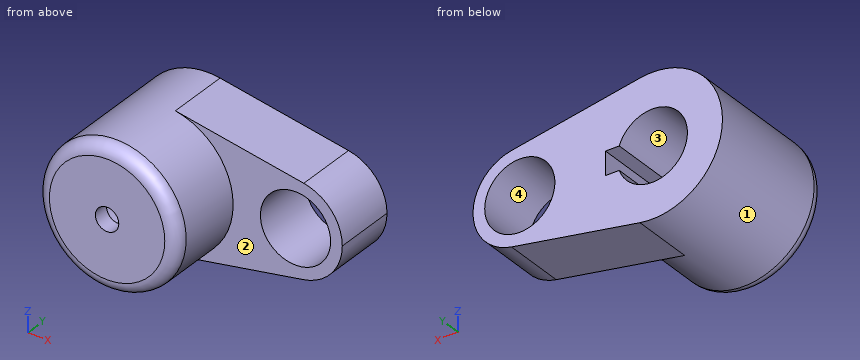
```python
from build123d import *

# Parameters (mm, degrees)
F0_R     = 14.2875
F1_DEPTH = 25.4
F2_DEPTH = 50.8
F3_R     = 28.575
F3_R_2   = 4.7625
F4_DEPTH = 6.35
F5_R     = 5.08


with BuildPart() as f1:
    # F0 (on Front) → F1 (new body)
    with BuildSketch(Plane.XZ):
        with BuildLine():
            ThreePointArc((5.0426470588, -28.1265414802), (21.9160245563, -18.3362616868), (28.575, 0))
            ThreePointArc((28.575, 0), (21.9160245563, 18.3362616868), (5.0426470588, 28.1265414802))
            ThreePointArc((5.0426470588, 28.1265414802), (-28.575, 0), (5.0426470588, -28.1265414802))
        make_face()
        with BuildLine():
            ThreePointArc((-13.4703841816, 4.7625), (0, 14.2875), (13.4703841816, 4.7625))
            Line((13.4703841816, 4.7625), (19.05, 4.7625))
            Line((19.05, 4.7625), (19.05, -4.7625))
            Line((19.05, -4.7625), (13.4703841816, -4.7625))
            ThreePointArc((13.4703841816, -4.7625), (0, -14.2875), (-13.4703841816, -4.7625))
            Line((-13.4703841816, -4.7625), (-19.05, -4.7625))
            Line((-19.05, -4.7625), (-19.05, 4.7625))
            Line((-19.05, 4.7625), (-13.4703841816, 4.7625))
        make_face(mode=Mode.SUBTRACT)
        with BuildLine():
            ThreePointArc((5.0426470588, 28.1265414802), (21.9160245563, 18.3362616868), (28.575, 0))
            ThreePointArc((28.575, 0), (21.9160245563, -18.3362616868), (5.0426470588, -28.1265414802))
            Line((5.0426470588, -28.1265414802), (57.3367647059, -18.7510276535))
            ThreePointArc((57.3367647059, -18.7510276535), (34.925, 0), (57.3367647059, 18.7510276535))
            Line((57.3367647059, 18.7510276535), (5.0426470588, 28.1265414802))
        make_face()
        with BuildLine():
            ThreePointArc((73.025, 0), (68.5856830375, 12.2241744579), (57.3367647059, 18.7510276535))
            ThreePointArc((57.3367647059, 18.7510276535), (34.925, 0), (57.3367647059, -18.7510276535))
            ThreePointArc((57.3367647059, -18.7510276535), (68.5856830375, -12.2241744579), (73.025, 0))
        make_face()
        with Locations((53.975, 0)):
            Circle(F0_R, mode=Mode.SUBTRACT)
    extrude(amount=F1_DEPTH)

    # F0 (on Front) → F2 (join)
    with BuildSketch(Plane.XZ):
        with BuildLine():
            ThreePointArc((5.0426470588, -28.1265414802), (21.9160245563, -18.3362616868), (28.575, 0))
            ThreePointArc((28.575, 0), (21.9160245563, 18.3362616868), (5.0426470588, 28.1265414802))
            ThreePointArc((5.0426470588, 28.1265414802), (-28.575, 0), (5.0426470588, -28.1265414802))
        make_face()
        with BuildLine():
            ThreePointArc((-13.4703841816, 4.7625), (0, 14.2875), (13.4703841816, 4.7625))
            Line((13.4703841816, 4.7625), (19.05, 4.7625))
            Line((19.05, 4.7625), (19.05, -4.7625))
            Line((19.05, -4.7625), (13.4703841816, -4.7625))
            ThreePointArc((13.4703841816, -4.7625), (0, -14.2875), (-13.4703841816, -4.7625))
            Line((-13.4703841816, -4.7625), (-19.05, -4.7625))
            Line((-19.05, -4.7625), (-19.05, 4.7625))
            Line((-19.05, 4.7625), (-13.4703841816, 4.7625))
        make_face(mode=Mode.SUBTRACT)
        with BuildLine():
            ThreePointArc((-13.4703841816, -4.7625), (-14.2875, 0), (-13.4703841816, 4.7625))
            Line((-13.4703841816, 4.7625), (-19.05, 4.7625))
            Line((-19.05, 4.7625), (-19.05, -4.7625))
            Line((-19.05, -4.7625), (-13.4703841816, -4.7625))
        make_face()
    extrude(amount=F2_DEPTH)

    # F3 (on face) → F4 (join)
    with BuildSketch(Plane.XZ.offset(50.8)):
        Circle(F3_R)
        Circle(F3_R_2, mode=Mode.SUBTRACT)
    extrude(amount=F4_DEPTH)

    # F5
    f5_edges = [f1.edges().sort_by_distance(p)[0] for p in [
        (-28.575, -57.15, 0),
    ]]
    fillet(f5_edges, radius=F5_R)


solid = f1.part
```
Geometry check sheet. Reference: the model listing, model coordinates, mm. Face numbers are marked on the shaded views. Give positions to 0.01 mm unless a question says otherwise; leave off trailing zeros. Order: outer loops, then holes, each group sorted by start corner. A loop starts at its lowest first (then second) coordinate and runs counter-clockwise, first axis right, second up. Notation, with made-up numbers: (77, -33) - (118, -33) arc R12 ccw to (118, -10) - close; hole circle Ø8 at (16.5, 83). An arc over 180 degrees is marked (long way). Answer in a Markdown table with one row per item. Add a question column.
Q1. Material ranges on probe 1 along Z at (x, y) = (0, -11) (1 decimal); probe 2 along X at (y, z) = (-3, 1.5); probe 3 along X at (y, z) = (-15, -1), recorded low to high. Write a range as from..to.
Q2. Gauge pin test, flat ends, axial feed: pin 1 (10 mm diameter, centred on x = 60.5, z = 1.5, fed in from +Y); pin 2 (5 mm diameter, centred on x = 25.5, y = -51, fed in from -Z); pin 3 (6 mm diameter, centred on x = 16, y = -37.5, fed in from +Z); pin 4 (14.5 mm diameter, centred on x = -3.5, z = -0.5, fed in from +Y). Record the tip position at first contact, or that the pin passes through.
Q3. Cross-section at D-D, the plane x = 46.5. Enter the section's corners in (y, z).
Q4. Mould release check, pull along Z, two halves, no side actions. Record for the marked faces 1, 2, 3 and 4: pulls with the +Z half, pulls with the -Z half, needs draft (parallel to the pull), parting line crosses it, or undercut.
Q5. Cross-section at B-B, the plane y = -9. Count the separate pieces of the cut face and the enclosed holes in it, then the cut area to 3 significant figures.
Check values:
| question | item | result |
|---|---|---|
| 1 | probe 1 | z = -28.6..-14.3, 14.3..28.6 |
| 1 | probe 2 | x = -28.54..-14.21, 19.05..39.77, 68.18..72.97 |
| 1 | probe 3 | x = -28.56..-14.25, 19.05..39.72, 68.23..73 |
| 2 | pin 1 | passes through |
| 2 | pin 2 | stops at z = -16.96 |
| 2 | pin 3 | stops at z = 25.45 |
| 2 | pin 4 | stops at y = -50.8 |
| 3 | outline | (-25.4, -20.69) - (0, -20.69) - (0, -12.18) - (-25.4, -12.18) - close; (-25.4, 12.18) - (0, 12.18) - (0, 20.69) - (-25.4, 20.69) - close |
| 4 | face 1 | parting line crosses it |
| 4 | face 2 | needs draft |
| 4 | face 3 | undercut |
| 4 | face 4 | undercut |
| 5 | separate pieces | 1 |
| 5 | enclosed holes | 2 |
| 5 | area | 3,130 mm^2 |
